Part model, mm, in its own coordinate system. A direction names the side the tool comes from. Coordinates: 2 decimals unless noted, no trailing zeros. Loops run counter-clockwise (first coordinate to the right, second up) from the corner with the lowest first, then second, coordinate; pieces in that order, holes last. Notation, with made-up numbers: (14, -27.75) - (32, -27.75) arc R19 ccw to (32, 6.25) - close; hole circle Ø11 at (69.25, -8). An arc over 180 degrees is marked (long way). Use a Markdown table: item, result. Add a question column.
1) Drop flat-ended pins along their axis: P1, Ø1.8, axis at x = -20, y = 3.5, coming from the +Z side; P2, Ø1.8, axis at y = 3, z = 66.5, coming from the -X side. Give the stop position or say it passes through.
2) Probe probe 1 along X at (y, z) = (4.5, 56.75); probe 2 along X at (y, z) = (2.1, 63.25); probe 3 along Z at (x, y) = (-12, 2.95). List the from-to ranges inside material, lowest first. Write a range as [from, to].
3) Tool access for faces 4 (the face through (21, 3, 65)), 5 (the face through (-16, 3, 65)), 6 (the face through (-4, 3, 65)), 7 (the face through (-4, 3, 56)): list every direction of +Z, -Z, +X, -X, +Y, -Y with a clear straight run to the whole face (end or side of a thin tool).
4) Pull direction Z, two halves, no side cores. Call faces 1 (the face through (3, 3, 62.081)), 2 (the face through (15, 3, 53.081)), 3 (the face through (9, 3, 65)): +Z half, -Z half, draft (parallel to the pull), parting line (faces both ways), or undercut.
5) Band-saw the part on A-A (z = 58.25). Give the cut face in (x, y).
6) Band-saw the part on B-B (x = 12.5). Give the cut face in (y, z), plus the area to 3 significant figures.
7) Band-saw the part on C-C (y = 2). Give the cut face in (x, z).
8) Band-saw the part on D-D (x = -18). Give the cut face in (y, z).
Autodesk Inventor part; units mm, degrees
ref_plane "YZ Plane" through (0, 0, 0) normal (1, 0, 0) x (0, 1, 0)
ref_plane "XZ Plane" through (0, 0, 0) normal (0, 1, 0) x (-1, 0, 0)
ref_plane "XY Plane" through (0, 0, 0) normal (0, 0, 1) x (1, 0, 0)
sketch "Sketch1" plane through (0, 0, 0) normal (0, 1, 0) x (-1, 0, 0)
  line L0 (27.5, 50.0814) -> (27.5, 62.0814)
  line L1 (-32.5, 62.0814) -> (-32.5, 50.0814)
  line L2 (-32.5, 50.0814) -> (-2.5, 50.0814)
  line L3 (-2.5, 50.0814) -> (-2.5, 62.0814) construction
  line L4 (-32.5, 56.0814) -> (-2.5, 56.0814) construction
  line L5 (-32.5, 62.0814) -> (27.5, 62.0814)
  line L6 (-21, 62.0814) -> (-9, 62.0814)
  line L7 (-9, 62.0814) -> (-9, 68.0814)
  line L8 (-9, 68.0814) -> (-21, 68.0814)
  line L9 (-21, 68.0814) -> (-21, 62.0814)
  line L10 (16, 62.0814) -> (4, 62.0814)
  line L11 (4, 62.0814) -> (4, 68.0814)
  line L12 (4, 68.0814) -> (16, 68.0814)
  line L13 (16, 68.0814) -> (16, 62.0814)
  line L14 (-2.5, 56.0814) -> (27.5, 56.0814) construction
  line L15 (-2.5, 50.0814) -> (27.5, 50.0814)
  line L16 (-9, 59.0814) -> (-21, 59.0814)
  line L17 (-21, 59.0814) -> (-21, 53.0814)
  line L18 (-21, 53.0814) -> (-9, 53.0814)
  line L19 (-9, 53.0814) -> (-9, 59.0814)
  line L20 (-9, 59.0814) -> (-21, 53.0814) construction
  line L21 (-21, 59.0814) -> (-9, 53.0814) construction
  line L22 (4, 59.0814) -> (16, 59.0814)
  line L23 (16, 59.0814) -> (16, 53.0814)
  line L24 (16, 53.0814) -> (4, 53.0814)
  line L25 (4, 53.0814) -> (4, 59.0814)
  line L26 (4, 59.0814) -> (16, 53.0814) construction
  line L27 (16, 59.0814) -> (4, 53.0814) construction
  point P0 (-15, 56.0814)
  point P1 (10, 56.0814)
  dimension "d0" = 60
  dimension "d1" = 12
  dimension "d18" = 12
  dimension "d19" = 6
  dimension "d20" = 18.5
  dimension "d21" = 12
  dimension "d22" = 6
  dimension "d23" = 3
extrude "Extrusion1" add sketch "Sketch1" along normal blind 6
sketch "Sketch3" plane through (0, 0, 0) normal (0, 1, 0) x (-1, 0, 0)
  line L0 (4, 62.0814) -> (-9, 62.0814) construction
  line L1 (-2.5, 62.0814) -> (-2.5, 50.0814) construction
  line L2 (-32.5, 50.0814) -> (27.5, 50.0814) construction
  line L3 (8.5, 50.0814) -> (2.5, 50.0814)
  line L4 (2.5, 50.0814) -> (2.5, 44.0814)
  line L5 (2.5, 44.0814) -> (8.5, 44.0814)
  line L6 (8.5, 44.0814) -> (8.5, 50.0814)
  line L7 (8.5, -0.9186) -> (2.5, -0.9186)
  line L8 (2.5, -0.9186) -> (2.5, -6.9186)
  line L9 (2.5, -6.9186) -> (8.5, -6.9186)
  line L10 (8.5, -6.9186) -> (8.5, -0.9186)
  line L11 (8.5, 35.0814) -> (-9.5, 35.0814)
  line L12 (-9.5, 35.0814) -> (-9.5, 23.0814)
  line L13 (-9.5, 13.0814) -> (8.5, 13.0814)
  line L14 (8.5, 13.0814) -> (8.5, 23.0814)
  line L15 (-13, 35.0814) -> (12, 35.0814)
  line L16 (8.5, 23.0814) -> (-9.5, 23.0814)
  line L17 (1.5, 35.0814) -> (-5.5, 35.0814)
  line L18 (-5.5, 35.0814) -> (-5.5, 40.0814)
  line L19 (-5.5, 40.0814) -> (1.5, 40.0814)
  line L20 (1.5, 40.0814) -> (1.5, 35.0814)
  line L21 (-9.5, 23.0814) -> (-9.5, 13.0814)
  line L22 (8.5, 23.0814) -> (8.5, 35.0814)
  point P0 (0, 0)
  dimension "d37" = 6
  dimension "d38" = 6
  dimension "d39" = 6
  dimension "d43" = 12
  dimension "d44" = 45
  dimension "d45" = 5
  dimension "d46" = 18
  dimension "d47" = 22
  dimension "d53" = 9
  dimension "d58" = 7
  dimension "d59" = 5
  dimension "d60" = 1
extrude "Extrusion3" cut sketch "Sketch3" along normal through all
properties part number "thumper-bumper-sidewall2-v3"
Answer block:
| question | item | result |
|---|---|---|
| 1 | P1 | z = 62.08 |
| 1 | P2 | x = -16 |
| 2 | probe 1 | [-27.5, -16], [-4, 9], [21, 32.5] |
| 2 | probe 2 | [-16, -4], [9, 21] |
| 2 | probe 3 | [50.08, 53.08], [59.08, 68.08] |
| 3 | face 4 | +Z, +X, +Y, -Y |
| 3 | face 5 | +Z, -X, +Y, -Y |
| 3 | face 6 | +Z, +Y, -Y |
| 3 | face 7 | +Y, -Y |
| 4 | face 1 | +Z half |
| 4 | face 2 | undercut |
| 4 | face 3 | draft |
| 5 | outline | (-27.5, 0) - (-16, 0) - (-16, 6) - (-27.5, 6) - close; (-4, 0) - (9, 0) - (9, 6) - (-4, 6) - close; (21, 0) - (32.5, 0) - (32.5, 6) - (21, 6) - close |
| 6 | outline | (0, 50.08) - (6, 50.08) - (6, 53.08) - (0, 53.08) - close; (0, 59.08) - (6, 59.08) - (6, 68.08) - (0, 68.08) - close |
| 6 | area | 72.0 mm2 |
| 7 | outline | (-27.5, 50.08) - (32.5, 50.08) - (32.5, 62.08) - (21, 62.08) - (21, 68.08) - (9, 68.08) - (9, 62.08) - (-4, 62.08) - (-4, 68.08) - (-16, 68.08) - (-16, 62.08) - (-27.5, 62.08) - close; hole (-16, 53.08) - (-4, 53.08) - (-4, 59.08) - (-16, 59.08) - close; hole (9, 53.08) - (21, 53.08) - (21, 59.08) - (9, 59.08) - close |
| 8 | outline | (0, 50.08) - (6, 50.08) - (6, 62.08) - (0, 62.08) - close |
